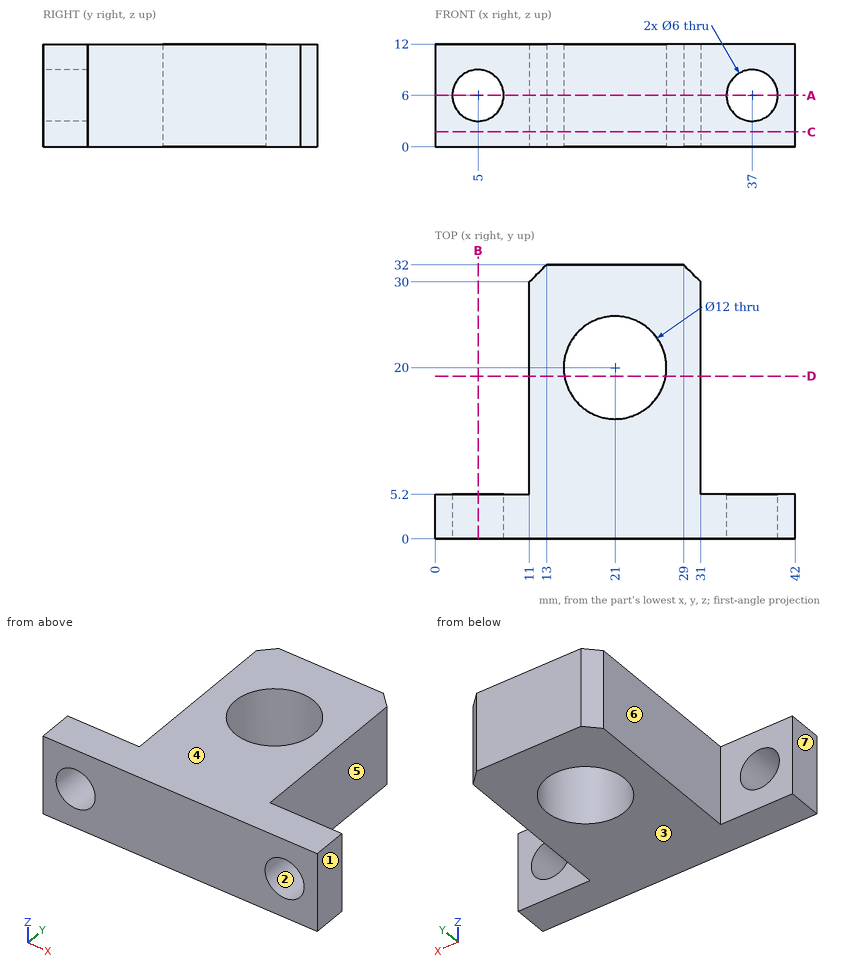
Could you check a few things on this drawing? It's one solid part, dimensions in mm from its lowest x, y, z. A direction names the side the tool comes from. Round coordinates to 2 decimals unless told otherwise and drop trailing zeros. Loops run counter-clockwise (first coordinate to the right, second up) from the corner with the lowest first, then second, coordinate; pieces in that order, holes last. Notation, with made-up numbers: M 49.25,40 L 72.25,40 A22 ccw 72.25,73 Z; hole C 28.25,86 d5. An arc over 180 degrees is marked long. Write item = value, one per line. Start each with the question number.
(1) Suppose I cut it at D-D on y = 19. Write out the boundary of the cut face in (x, z).
(2) I need wall thicknesses on line 1 along Y through (x, z) = (21, 4.75); line 2 along Z through (x, y) = (5, 3.35); line 3 along X through (y, z) = (3, 5.5). Which ranges of each line are inside material? Lowest first, please.
(3) If we mould it in two halves opening along Z, with no side actions, what happens to the marked faces 1, 2, 3 and 4? For each: released by +Z, released by -Z, zero draft, split by the parting line, or undercut.
(4) Suppose I cut it at C-C on z = 1.75. Write out the boundary of the cut face in (x, y).
(5) Suppose I cut it at B-B on x = 5. Write out the boundary of the cut face in (y, z).
(6) Suppose I cut it at A-A on z = 6. Write out the boundary of the cut face in (x, y), plus the area to 3 significant figures.
(7) Which directions (+Z, -Z, +X, -X, +Y, -Y) give clear straight access to the entire face, cutting with the end or side of a thin tool? Please do the marked faces 5, 6 and 7.
(8) I'm going to push flat-ended pins straight in: P1, Ø1, axis at y = 20, z = 7.5, coming from the +X side; P2, Ø4, axis at x = 13.5, y = 17, coming from the -Z side; P3, Ø1.5, axis at y = 16, z = 2.5, coming from the -X side. Where does each tip first touch, or does it pass through?
Answer block:
q1.outline = M 11,0 L 15.08,0 L 15.08,12 L 11,12 Z; M 26.92,0 L 31,0 L 31,12 L 26.92,12 Z
q2.line_1 = 0 to 14, 26 to 32
q2.line_2 = 0 to 3, 9 to 12
q2.line_3 = 0 to 2.04, 7.96 to 34.04, 39.96 to 42
q3.face_1 = zero draft
q3.face_2 = undercut
q3.face_3 = released by -Z
q3.face_4 = released by +Z
q4.outline = M 0,0 L 42,0 L 42,5.2 L 31,5.2 L 31,30 L 29,32 L 13,32 L 11,30 L 11,5.2 L 0,5.2 Z; hole C 21,20 d12
q5.outline = M 0,0 L 5.2,0 L 5.2,3 L 0,3 Z; M 0,9 L 5.2,9 L 5.2,12 L 0,12 Z
q6.outline = M 0,0 L 2,0 L 2,5.2 L 0,5.2 Z; M 8,0 L 34,0 L 34,5.2 L 31,5.2 L 31,30 L 29,32 L 13,32 L 11,30 L 11,5.2 L 8,5.2 Z; M 40,0 L 42,0 L 42,5.2 L 40,5.2 Z; hole C 21,20 d12
q6.area = 575 mm²
q7.face_5 = +Z, -Z, +X, +Y
q7.face_6 = +Z, -Z, -X, +Y
q7.face_7 = +Z, -Z, -X, +Y, -Y
q8.P1 = 31
q8.P2 = 0
q8.P3 = 11
